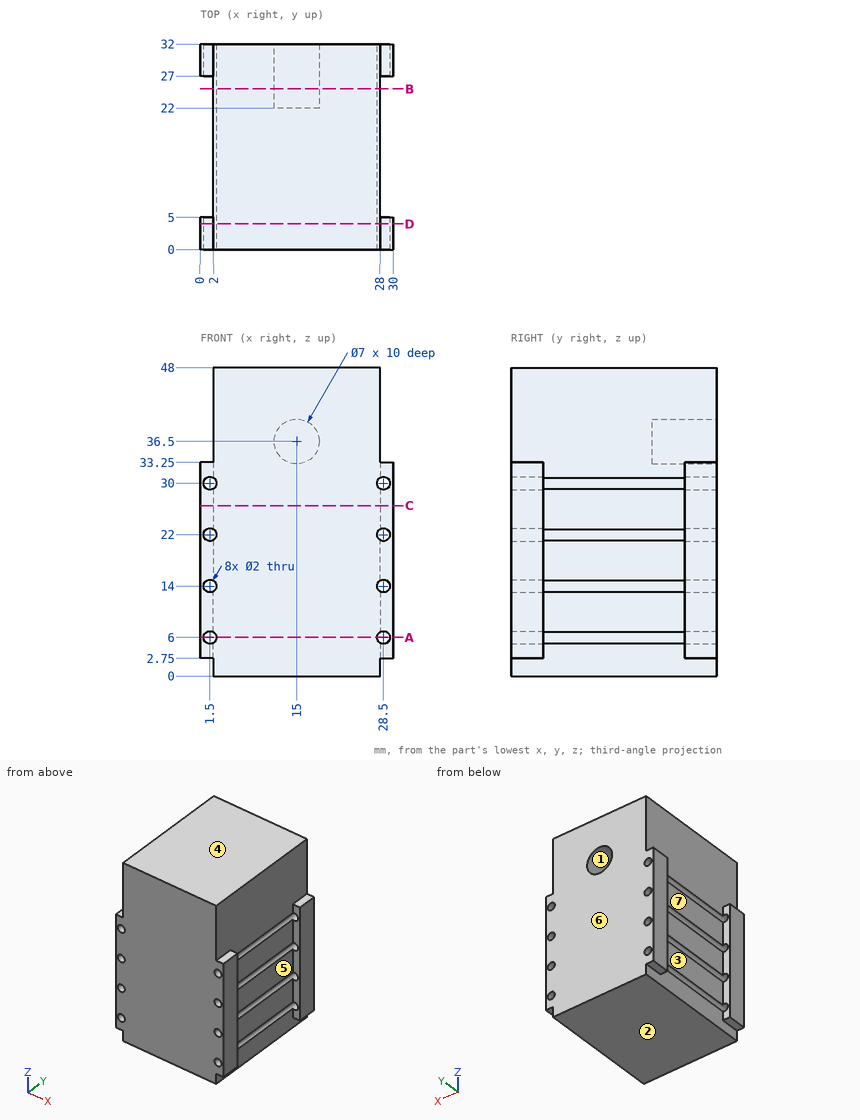
Part print with two shaded views. Sizes in mm from the minimum x, y, z corner. A direction names the side the tool comes from. Round coordinates to 2 decimals unless told otherwise and drop trailing zeros. Write each loop counter-clockwise with the first axis right and the second up, starting at its lowest first coordinate (ties: lowest second). Pieces come first, ordered by that corner, then holes. Notation, with made-up numbers: (84.5, 22) -> (139.5, 22) arc R13 cw to (139.5, 41) -> close; hole circle Ø8 at (-38.5, 59.5). An arc over 180 degrees is marked (long way). Put each result on its own line as item: value.
Item 1: Slice it at A-A, the plane z = 6. Give the cut face in (x, y), plus the area to 3 significant figures.
Here are the results:
outline: (0, 0) -> (0.5, 0) -> (0.5, 5) -> (0, 5) -> close; (0, 27) -> (0.5, 27) -> (0.5, 32) -> (0, 32) -> close; (2.5, 0) -> (27.5, 0) -> (27.5, 32) -> (2.5, 32) -> close; (29.5, 0) -> (30, 0) -> (30, 5) -> (29.5, 5) -> close; (29.5, 27) -> (30, 27) -> (30, 32) -> (29.5, 32) -> close
area: 810 mm^2
Item 2: Wall check: probe 1 along X at (y, z) = (18, 22); probe 2 along X at (y, z) = (9, 41.5); probe 3 along Y at (x, z) = (28.5, 26.5). Give the ranges that are in metal, low to high. Write a range as from..to.
Here are the results:
probe 1: x = 2.5..27.5
probe 2: x = 2..28
probe 3: y = 0..5, 27..32
Item 3: Flat gauge pins, fed straight in: P1, Ø2.5, axis at x = 28.5, z = 30, coming from the -Y side; P2, Ø8, axis at y = 22.5, z = 12, coming from the -X side; P3, Ø5, axis at y = 13.5, z = 42.5, coming from the +X side; P4, Ø2, axis at x = 0.5, y = 2.5, coming from the -Z side. Where does each tip first touch, or does it go through?
Here are the results:
P1: stops at y = 0
P2: stops at x = 2
P3: stops at x = 28
P4: stops at z = 2.75
Item 4: Tool access for the marked faces 5, 6 and 7: list every direction of +Z, -Z, +X, -X, +Y, -Y with a clear straight run to the whole face (end or side of a thin tool).
Here are the results:
face 5: +Z, -Z, +X
face 6: +Z, -Z, +X, -X, +Y
face 7: +Z, -Z, -X
Item 5: Slice it at C-C, the plane z = 26.5. Give the cut face in (x, y), plus the area to 3 significant figures.
Here are the results:
outline: (0, 0) -> (30, 0) -> (30, 5) -> (28, 5) -> (28, 27) -> (30, 27) -> (30, 32) -> (0, 32) -> (0, 27) -> (2, 27) -> (2, 5) -> (0, 5) -> close
area: 872 mm^2
Item 6: Two-plate mould, pull along Z, no slides. Class the marked faces 1, 2, 3 and 4: pulls with the +Z half, pulls with the -Z half, needs draft (parallel to the pull), parting line crosses it, or undercut.
Here are the results:
face 1: undercut
face 2: pulls with the -Z half
face 3: needs draft
face 4: pulls with the +Z half
Item 7: Slice it at B-B, the plane y = 25. Give the cut face in (x, z), plus the area to 3 significant figures.
Here are the results:
outline: (2, 0) -> (28, 0) -> (28, 5.13) arc R1 cw to (28, 6.87) -> (28, 13.13) arc R1 cw to (28, 14.87) -> (28, 21.13) arc R1 cw to (28, 22.87) -> (28, 29.13) arc R1 cw to (28, 30.87) -> (28, 48) -> (2, 48) -> (2, 30.87) arc R1 cw to (2, 29.13) -> (2, 22.87) arc R1 cw to (2, 21.13) -> (2, 14.87) arc R1 cw to (2, 13.13) -> (2, 6.87) arc R1 cw to (2, 5.13) -> close; hole circle Ø7 at (15, 36.5)
area: 1,200 mm^2
Item 8: Slice it at D-D, the plane y = 4. Count the separate pieces of the cut face and the enclosed holes in it, plus the area to 3 significant figures.
Here are the results:
separate pieces: 1
enclosed holes: 8
area: 1,340 mm^2
